Autodesk Inventor part; units mm, degrees
ref_plane "YZ Plane" through (0, 0, 0) normal (1, 0, 0) x (0, 1, 0)
ref_plane "XZ Plane" through (0, 0, 0) normal (0, 1, 0) x (-1, 0, 0)
ref_plane "XY Plane" through (0, 0, 0) normal (0, 0, 1) x (1, 0, 0)
sketch "Skizze1" plane through (0, 0, 0) normal (0, 1, 0) x (-1, 0, 0)
  circle A0 centre (0, 5) radius 1.05
  circle A1 centre (0, -5) radius 1.05
  line L0 (0, 5) -> (0, -5) construction
  line L1 (0, 5) -> (0, -5) construction
  line L2 (-4.05, 5) -> (-4.05, -5)
  line L3 (4.05, -5) -> (4.05, 5)
  arc A2 (4.05, 5) -> (-4.05, 5) centre (0, 5) ccw
  arc A3 (-4.05, -5) -> (4.05, -5) centre (0, -5) ccw
  point P0 (0, 0)
  point P1 (0, 0)
  point P2 (0, 0)
  dimension "d0" = 2.1
  dimension "d1" = 10
  dimension "d2" = 3
extrude "Extrusion1" add sketch "Skizze1" along normal blind 3
sketch "Skizze2" plane through (0, 3, 0) normal (0, 1, 0) x (1, 0, 0)
  circle A0 centre (0, 5) radius 1.05
  line L0 (2.3094, 5) -> (1.1547, 3)
  line L1 (1.1547, 3) -> (-1.1547, 3)
  line L2 (-1.1547, 3) -> (-2.3094, 5)
  line L3 (-2.3094, 5) -> (-1.1547, 7)
  line L4 (-1.1547, 7) -> (1.1547, 7)
  line L5 (1.1547, 7) -> (2.3094, 5)
  circle A1 centre (0, -5) radius 1.05
  line L6 (1.1547, -3) -> (2.3094, -5)
  line L7 (2.3094, -5) -> (1.1547, -7)
  line L8 (1.1547, -7) -> (-1.1547, -7)
  line L9 (-1.1547, -7) -> (-2.3094, -5)
  line L10 (-2.3094, -5) -> (-1.1547, -3)
  line L11 (-1.1547, -3) -> (1.1547, -3)
  point P0 (0, 0)
  dimension "d5" = 4
extrude "Extrusion2" cut sketch "Skizze2" against normal blind 1.6
sketch "Skizze3" plane through (0, 0, 0) normal (0, -1, 0) x (1, 0, 0)
  circle A0 centre (0, -5) radius 1.05
  circle A1 centre (0, -5) radius 1.5
  circle A2 centre (0, 5) radius 1.05
  circle A3 centre (0, 5) radius 1.5
  point P0 (0, 0)
  dimension "d8" = 3
extrude "Extrusion3" add sketch "Skizze3" along normal blind 1.5
properties part number "_3D-Druck"
Could you check a few things on this model? Use its own coordinates, in mm. A direction names the side the tool comes from. Round coordinates to 2 decimals unless told otherwise and drop trailing zeros. Loops run counter-clockwise (first coordinate to the right, second up) from the corner with the lowest first, then second, coordinate; pieces in that order, holes last. Notation, with made-up numbers: (13, 49.5) -> (69, 49.5) arc R31 cw to (69, 79.5) -> close; hole circle Ø11 at (-9, -4). An arc over 180 degrees is marked (long way). One line per question, with ' | ' between items.
(1) If we section it at C-C on z = -4.5: List the corners of the cut face in (x, y) for me.
Model answer:
outline: (-4.05, 0) -> (-1.41, 0) -> (-1.41, -1.5) -> (-0.92, -1.5) -> (-0.92, 1.4) -> (-2.02, 1.4) -> (-2.02, 3) -> (-4.05, 3) -> close; (0.92, -1.5) -> (1.41, -1.5) -> (1.41, 0) -> (4.05, 0) -> (4.05, 3) -> (2.02, 3) -> (2.02, 1.4) -> (0.92, 1.4) -> close
(2) If we section it at D-D on y = -0.4: List the corners of the cut face in (x, z) for me.
Model answer:
outline: circle Ø3 at (0, -5); circle Ø3 at (0, 5); hole circle Ø2.1 at (0, -5); hole circle Ø2.1 at (0, 5)
(3) If I drill on probe 1 along Z at (x, y) = (0, -0.3); probe 2 along Z at (x, y) = (0, 2.8); probe 3 along Z at (x, y) = (0, 1.1), over which ranges is the centre line in solid material (lowest first)?
Model answer:
probe 1: z = -6.5 to -6.05, -3.95 to -3.5, 3.5 to 3.95, 6.05 to 6.5 | probe 2: z = -9.05 to -7, -3 to 3, 7 to 9.05 | probe 3: z = -9.05 to -6.05, -3.95 to 3.95, 6.05 to 9.05
(4) For faces 1 (the face through (-0.195, -0.74, 3.513)), 2 (the face through (0.09, 1.48, 9.05)), 3 (the face through (1.74, 2.21, -4.01)), which set-ups out of +Z, -Z, +X, -X, +Y, -Y let a thin tool reach every point of the face, with its end or its side?
Model answer:
face 1: -Y | face 2: +Z, +Y, -Y | face 3: +Y
(5) For pin 1 Ø2 at (y, z) = (2.5, 6.5) entering from +X; pin 2 Ø3.5 at (x, z) = (0, 5) entering from -Y; pin 3 Ø1 at (x, z) = (-2, 1.5) entering from -Y; pin 4 Ø2 at (x, z) = (1, 5) entering from +Y, each with a flat end and sliding along its axis, tell me the tip position at first contact or that it passes through.
Model answer:
pin 1: stops at x = 4.02 | pin 2: stops at y = -1.5 | pin 3: stops at y = 0 | pin 4: stops at y = 1.4
(6) If we section it at B-B on x = 0: List the corners of the cut face in (y, z) for me, and give its area (3 significant figures).
Model answer:
outline: (-1.5, -6.5) -> (0, -6.5) -> (0, -9.05) -> (3, -9.05) -> (3, -7) -> (1.4, -7) -> (1.4, -6.05) -> (-1.5, -6.05) -> close; (-1.5, -3.95) -> (1.4, -3.95) -> (1.4, -3) -> (3, -3) -> (3, 3) -> (1.4, 3) -> (1.4, 3.95) -> (-1.5, 3.95) -> (-1.5, 3.5) -> (0, 3.5) -> (0, -3.5) -> (-1.5, -3.5) -> close; (-1.5, 6.05) -> (1.4, 6.05) -> (1.4, 7) -> (3, 7) -> (3, 9.05) -> (0, 9.05) -> (0, 6.5) -> (-1.5, 6.5) -> close | area: 38.3 mm^2
(7) Thinking about a two-plate mould opening in X: for faces 4 (the face through (4.05, 1, 0)), 5 (the face through (0, 2, -3)), 6 (the face through (-1.74, 2.21, -5.99)), 7 (the face through (0, 3, 0)), which applies, released by +X, released by -X, zero draft, split by the parting line, or undercut?
Model answer:
face 4: released by +X | face 5: undercut | face 6: undercut | face 7: zero draft
(8) If we section it at A-A on y = 2.3: List the corners of the cut face in (x, z) for me, and give its area (3 significant figures).
Model answer:
outline: (-4.05, -5) arc R4.05 ccw to (4.05, -5) -> (4.05, 5) arc R4.05 ccw to (-4.05, 5) -> close; hole (-2.31, -5) -> (-1.15, -7) -> (1.15, -7) -> (2.31, -5) -> (1.15, -3) -> (-1.15, -3) -> close; hole (-2.31, 5) -> (-1.15, 3) -> (1.15, 3) -> (2.31, 5) -> (1.15, 7) -> (-1.15, 7) -> close | area: 105 mm^2
